from build123d import *

# Parameters (mm, degrees)
F0_R     = 2.54
F1_DEPTH = 4.064
F2_DEPTH = 3.302
F3_DEPTH = 2.54
F0_R_2   = 27.94
F4_DEPTH = 1.778


with BuildPart() as f1:
    # F0 (on Front) → F1 (new body)
    with BuildSketch(Plane.XZ):
        with BuildLine():
            ThreePointArc((5.819871, -2.54), (6.216055, -1.297366), (6.35, 0))
            ThreePointArc((6.35, 0), (6.216055, 1.297366), (5.819871, 2.54))
            ThreePointArc((5.819871, 2.54), (4.490128, 4.490128), (2.54, 5.819871))
            ThreePointArc((2.54, 5.819871), (0, 6.35), (-2.54, 5.819871))
            ThreePointArc((-2.54, 5.819871), (-4.490128, 4.490128), (-5.819871, 2.54))
            ThreePointArc((-5.819871, 2.54), (-6.35, 0), (-5.819871, -2.54))
            ThreePointArc((-5.819871, -2.54), (-4.490128, -4.490128), (-2.54, -5.819871))
            ThreePointArc((-2.54, -5.819871), (0, -6.35), (2.54, -5.819871))
            ThreePointArc((2.54, -5.819871), (4.490128, -4.490128), (5.819871, -2.54))
        make_face()
        Circle(F0_R, mode=Mode.SUBTRACT)
        with BuildLine():
            ThreePointArc((-5.819871, -2.54), (-6.35, 0), (-5.819871, 2.54))
            Line((-5.819871, 2.54), (-8.519419, 2.54))
            ThreePointArc((-8.519419, 2.54), (-8.89, 0), (-8.519419, -2.54))
            Line((-8.519419, -2.54), (-5.819871, -2.54))
        make_face()
        with BuildLine():
            ThreePointArc((5.819871, 2.54), (6.216055, 1.297366), (6.35, 0))
            ThreePointArc((6.35, 0), (6.216055, -1.297366), (5.819871, -2.54))
            Line((5.819871, -2.54), (8.519419, -2.54))
            ThreePointArc((8.519419, -2.54), (8.796867, -1.283446), (8.89, 0))
            ThreePointArc((8.89, 0), (8.796867, 1.283446), (8.519419, 2.54))
            Line((8.519419, 2.54), (5.819871, 2.54))
        make_face()
    extrude(amount=F1_DEPTH)

    # F0 (on Front) → F2 (join)
    with BuildSketch(Plane.XZ):
        with BuildLine():
            ThreePointArc((12.443408, -2.54), (12.635689, -1.276464), (12.7, 0))
            ThreePointArc((12.7, 0), (12.635689, 1.276464), (12.443408, 2.54))
            ThreePointArc((12.443408, 2.54), (8.980256, 8.980256), (2.54, 12.443408))
            ThreePointArc((2.54, 12.443408), (0, 12.7), (-2.54, 12.443408))
            ThreePointArc((-2.54, 12.443408), (-8.980256, 8.980256), (-12.443408, 2.54))
            ThreePointArc((-12.443408, 2.54), (-12.7, 0), (-12.443408, -2.54))
            ThreePointArc((-12.443408, -2.54), (-8.980256, -8.980256), (-2.54, -12.443408))
            ThreePointArc((-2.54, -12.443408), (0, -12.7), (2.54, -12.443408))
            ThreePointArc((2.54, -12.443408), (8.980256, -8.980256), (12.443408, -2.54))
        make_face()
        with BuildLine():
            ThreePointArc((2.54, 8.519419), (6.286179, 6.286179), (8.519419, 2.54))
            ThreePointArc((8.519419, 2.54), (8.796867, 1.283446), (8.89, 0))
            ThreePointArc((8.89, 0), (8.796867, -1.283446), (8.519419, -2.54))
            ThreePointArc((8.519419, -2.54), (6.286179, -6.286179), (2.54, -8.519419))
            ThreePointArc((2.54, -8.519419), (0, -8.89), (-2.54, -8.519419))
            ThreePointArc((-2.54, -8.519419), (-6.286179, -6.286179), (-8.519419, -2.54))
            ThreePointArc((-8.519419, -2.54), (-8.89, 0), (-8.519419, 2.54))
            ThreePointArc((-8.519419, 2.54), (-6.286179, 6.286179), (-2.54, 8.519419))
            ThreePointArc((-2.54, 8.519419), (0, 8.89), (2.54, 8.519419))
        make_face(mode=Mode.SUBTRACT)
        with BuildLine():
            Line((2.54, -15.670483), (2.54, -12.443408))
            ThreePointArc((2.54, -12.443408), (0, -12.7), (-2.54, -12.443408))
            Line((-2.54, -12.443408), (-2.54, -15.670483))
            ThreePointArc((-2.54, -15.670483), (0, -15.875), (2.54, -15.670483))
        make_face()
        with BuildLine():
            ThreePointArc((-2.54, 12.443408), (0, 12.7), (2.54, 12.443408))
            Line((2.54, 12.443408), (2.54, 15.670483))
            ThreePointArc((2.54, 15.670483), (0, 15.875), (-2.54, 15.670483))
            Line((-2.54, 15.670483), (-2.54, 12.443408))
        make_face()
    extrude(amount=F2_DEPTH)

    # F0 (on Front) → F3 (join)
    with BuildSketch(Plane.XZ):
        with BuildLine():
            ThreePointArc((20.160625, -2.54), (20.280117, -1.272498), (20.32, 0))
            ThreePointArc((20.32, 0), (20.280117, 1.272498), (20.160625, 2.54))
            ThreePointArc((20.160625, 2.54), (14.36841, 14.36841), (2.54, 20.160625))
            ThreePointArc((2.54, 20.160625), (0, 20.32), (-2.54, 20.160625))
            ThreePointArc((-2.54, 20.160625), (-14.36841, 14.36841), (-20.160625, 2.54))
            ThreePointArc((-20.160625, 2.54), (-20.32, 0), (-20.160625, -2.54))
            ThreePointArc((-20.160625, -2.54), (-14.36841, -14.36841), (-2.54, -20.160625))
            ThreePointArc((-2.54, -20.160625), (0, -20.32), (2.54, -20.160625))
            ThreePointArc((2.54, -20.160625), (14.36841, -14.36841), (20.160625, -2.54))
        make_face()
        with BuildLine():
            ThreePointArc((2.54, 15.670483), (11.22532, 11.22532), (15.670483, 2.54))
            ThreePointArc((15.670483, 2.54), (15.823788, 1.27411), (15.875, 0))
            ThreePointArc((15.875, 0), (15.823788, -1.27411), (15.670483, -2.54))
            ThreePointArc((15.670483, -2.54), (11.22532, -11.22532), (2.54, -15.670483))
            ThreePointArc((2.54, -15.670483), (0, -15.875), (-2.54, -15.670483))
            ThreePointArc((-2.54, -15.670483), (-11.22532, -11.22532), (-15.670483, -2.54))
            ThreePointArc((-15.670483, -2.54), (-15.875, 0), (-15.670483, 2.54))
            ThreePointArc((-15.670483, 2.54), (-11.22532, 11.22532), (-2.54, 15.670483))
            ThreePointArc((-2.54, 15.670483), (0, 15.875), (2.54, 15.670483))
        make_face(mode=Mode.SUBTRACT)
        with BuildLine():
            ThreePointArc((20.160625, 2.54), (20.280117, 1.272498), (20.32, 0))
            ThreePointArc((20.32, 0), (20.280117, -1.272498), (20.160625, -2.54))
            Line((20.160625, -2.54), (23.995943, -2.54))
            ThreePointArc((23.995943, -2.54), (24.096463, -1.271768), (24.13, 0))
            ThreePointArc((24.13, 0), (24.096463, 1.271768), (23.995943, 2.54))
            Line((23.995943, 2.54), (20.160625, 2.54))
        make_face()
        with BuildLine():
            ThreePointArc((-20.160625, -2.54), (-20.32, 0), (-20.160625, 2.54))
            Line((-20.160625, 2.54), (-23.995943, 2.54))
            ThreePointArc((-23.995943, 2.54), (-24.13, 0), (-23.995943, -2.54))
            Line((-23.995943, -2.54), (-20.160625, -2.54))
        make_face()
    extrude(amount=F3_DEPTH)

    # F0 (on Front) → F4 (join)
    with BuildSketch(Plane.XZ):
        Circle(F0_R_2)
        with BuildLine():
            ThreePointArc((2.54, 23.995943), (17.062487, 17.062487), (23.995943, 2.54))
            ThreePointArc((23.995943, 2.54), (24.096463, 1.271768), (24.13, 0))
            ThreePointArc((24.13, 0), (24.096463, -1.271768), (23.995943, -2.54))
            ThreePointArc((23.995943, -2.54), (17.062487, -17.062487), (2.54, -23.995943))
            ThreePointArc((2.54, -23.995943), (0, -24.13), (-2.54, -23.995943))
            ThreePointArc((-2.54, -23.995943), (-17.062487, -17.062487), (-23.995943, -2.54))
            ThreePointArc((-23.995943, -2.54), (-24.13, 0), (-23.995943, 2.54))
            ThreePointArc((-23.995943, 2.54), (-17.062487, 17.062487), (-2.54, 23.995943))
            ThreePointArc((-2.54, 23.995943), (0, 24.13), (2.54, 23.995943))
        make_face(mode=Mode.SUBTRACT)
    extrude(amount=F4_DEPTH)


solid = f1.part
Can you work these out from the model? Positions are in its coordinate system, mm. A direction names the side the tool comes from. Round coordinates to 2 decimals unless told otherwise and drop trailing zeros. Loops run counter-clockwise (first coordinate to the right, second up) from the corner with the lowest first, then second, coordinate; pieces in that order, holes last. Notation, with made-up numbers: (60, 30) - (105, 30) arc R21 ccw to (105, 39) - close; hole circle Ø11 at (-29, 14.5). An arc over 180 degrees is marked (long way). Use CSV: the item, a comma, the result in double quotes. Start each with the question number.
1) If we section it at D-D on y = -0.9: Count the separate pieces of the cut face and the enclosed holes in it, plus the area to 3 significant figures.
2) If we section it at C-C on x = 21.5: Write out the boundary of the cut face in (y, z), plus the area to 3 significant figures.
3) We'd pull the mould along X, two halves only. Please class faces 3 (the cylindrical face through (-3.64, -0.88, 27.7)), 4 (the flat face through (-2, -4.064, 2)), 5 (the cylindrical face through (-15.875, -1.252, -0.036)): released by +X, released by -X, zero draft, split by the parting line, or undercut.
4) If we section it at B-B on z = -14: Write out the boundary of the cut face in (x, y), plus the area to 3 significant figures.
5) For faces 1 (the flat face through (6, 0, 0)), 2 (the flat face through (-7, -2, 2.54)), which set-ups out of +Z, -Z, +X, -X, +Y, -Y let a thin tool reach every point of the face, with its end or its side?
6) For pin 1 Ø0.8 at (x, y) = (23, -1.5) entering from +Z; pin 2 Ø0.8 at (x, y) = (21.5, -1) entering from -Z; pin 3 Ø2 at (x, y) = (6.5, -3) entering from +Z, each with a flat end and sliding along its axis, tell me the tip position at first contact or that it passes through.
7) If we section it at A-A on x = 0: Write out the boundary of the cut face in (y, z) (3 decimals), plus the area to 3 significant figures.
8) Please list where these lines run through material, in increasing order: probe 1 along X at (y, z) = (-1.05, 13); probe 2 along Z at (x, y) = (-6.5, -2.5); probe 3 along X at (y, z) = (-3.2, -5). Write a range as [from, to].
Geometry results:
1,separate pieces,"1"
1,enclosed holes,"7"
1,area,"1,590 mm2"
2,outline,"(-2.54, -2.54) - (0, -2.54) - (0, 2.54) - (-2.54, 2.54) - close; (-1.78, -17.84) - (0, -17.84) - (0, -10.95) - (-1.78, -10.95) - close; (-1.78, 10.95) - (0, 10.95) - (0, 17.84) - (-1.78, 17.84) - close"
2,area,"37.4 mm2"
3,face 3,"split by the parting line"
3,face 4,"zero draft"
3,face 5,"undercut"
4,outline,"(-24.18, -1.78) - (-19.65, -1.78) - (-19.65, 0) - (-24.18, 0) - close; (-14.73, -2.54) - (-7.48, -2.54) - (-7.48, 0) - (-14.73, 0) - close; (-2.54, -3.3) - (2.54, -3.3) - (2.54, 0) - (-2.54, 0) - close; (7.48, -2.54) - (14.73, -2.54) - (14.73, 0) - (7.48, 0) - close; (19.65, -1.78) - (24.18, -1.78) - (24.18, 0) - (19.65, 0) - close"
4,area,"69.7 mm2"
5,face 1,"+Z, -Z, +X, -X, +Y"
5,face 2,"+Y, -Y"
6,pin 1,"stops at z = 16.43"
6,pin 2,"stops at z = -18.31"
6,pin 3,"stops at z = 19.53"
7,outline,"(-4.064, -6.35) - (0, -6.35) - (0, -2.54) - (-4.064, -2.54) - close; (-4.064, 2.54) - (0, 2.54) - (0, 6.35) - (-4.064, 6.35) - close; (-3.302, -15.875) - (-2.54, -15.875) - (-2.54, -20.32) - (0, -20.32) - (0, -8.89) - (-3.302, -8.89) - close; (-3.302, 8.89) - (0, 8.89) - (0, 20.32) - (-2.54, 20.32) - (-2.54, 15.875) - (-3.302, 15.875) - close; (-1.778, -27.94) - (0, -27.94) - (0, -24.13) - (-1.778, -24.13) - close; (-1.778, 24.13) - (0, 24.13) - (0, 27.94) - (-1.778, 27.94) - close"
7,area,"113 mm2"
8,probe 1,"x = [-24.73, -20.33], [-15.62, -9.11], [-2.54, 2.54], [9.11, 15.62], [20.33, 24.73]"
8,probe 2,"z = [-19.25, -14.48], [-10.91, -6.06], [-2.54, 2.54], [6.06, 10.91], [14.48, 19.25]"
8,probe 3,"x = [-11.67, -7.35], [-3.91, 3.91], [7.35, 11.67]"
